from build123d import *

# Parameters (mm, degrees)
BOSS_EXTRUDE1_DEPTH = 3.175
SKETCH3_W           = 7.9375
SKETCH3_H           = 228.6
CUT_EXTRUDE1_DEPTH  = 184.546857096
SKETCH4_R           = 3.175
CUT_EXTRUDE2_DEPTH  = 184.546857096
SKETCH5_R           = 1.5
CUT_EXTRUDE3_DEPTH  = 3.175


with BuildPart() as part:
    # Sketch2 → Boss-Extrude1 (new body)
    with BuildSketch(Plane.XY):
        Polygon((-92.075, 152.4), (-92.075, 108.857142857), (-88.9, 108.857142857), (-88.9, 65.314285714), (-92.075, 65.314285714), (-92.075, 21.771428571), (-88.9, 21.771428571), (-88.9, -21.771428571), (-92.075, -21.771428571), (-92.075, -65.314285714), (-88.9, -65.314285714), (-88.9, -108.857142857), (-92.075, -108.857142857), (-92.075, -152.4), (-53.34, -152.4), (-53.34, -158.75), (-17.78, -158.75), (-17.78, -152.4), (17.78, -152.4), (17.78, -158.75), (53.34, -158.75), (53.34, -152.4), (92.075, -152.4), (92.075, -108.857142857), (88.9, -108.857142857), (88.9, -65.314285714), (92.075, -65.314285714), (92.075, -21.771428571), (88.9, -21.771428571), (88.9, 21.771428571), (92.075, 21.771428571), (92.075, 65.314285714), (88.9, 65.314285714), (88.9, 108.857142857), (92.075, 108.857142857), (92.075, 152.4), align=None)
    extrude(amount=BOSS_EXTRUDE1_DEPTH)

    # Sketch3 → Cut-Extrude1 (cut, through all)
    with BuildSketch(Plane.XY.offset(3.175)):
        with Locations((0, 38.1)):
            Rectangle(SKETCH3_W, SKETCH3_H)
    extrude(amount=-CUT_EXTRUDE1_DEPTH, mode=Mode.SUBTRACT)

    # Sketch4 → Cut-Extrude2 (cut, through all)
    with BuildSketch(Plane.XY.offset(3.175)):
        with Locations((-50.8, -139.7)):
            Circle(SKETCH4_R)
    extrude(amount=-CUT_EXTRUDE2_DEPTH, mode=Mode.SUBTRACT)

    # Sketch5 → Cut-Extrude3 (cut)
    with BuildSketch(Plane.XY.offset(3.175)):
        with Locations((-73.025, 122.4)):
            Circle(SKETCH5_R)
        with Locations((-73.025, 106.65)):
            Circle(SKETCH5_R)
        with Locations((73.025, 122.4)):
            Circle(SKETCH5_R)
        with Locations((73.025, 106.65)):
            Circle(SKETCH5_R)
    extrude(amount=-CUT_EXTRUDE3_DEPTH, mode=Mode.SUBTRACT)


solid = part.part
Build history of the part. All positions in model axes, mm. Coordinates: 2 decimals unless noted, no trailing zeros. Order: outer loops, then holes, each group sorted by start corner. A loop starts at its lowest first (then second) coordinate and runs counter-clockwise, first axis right, second up. Notation, with made-up numbers: M 36,-8 L 93,-8 A37 cw 93,28 Z; hole C 31.25,-14.75 d3. An arc over 180 degrees is marked long. One line per question, with ' | ' between items. Start each with the question number.
Q1. Saw through at B-B (y = 86). List the corners of the cut face in (x, z) (3 decimals).
Q2. Flat gauge pins, fed straight in: pin 1 Ø1 at (x, z) = (91, 1.5) entering from -Y; pin 2 Ø1.8 at (x, y) = (73.025, 106.65) entering from +Z; pin 3 Ø1 at (y, z) = (16, 1) entering from -X; pin 4 Ø1.5 at (y, z) = (73.5, 2) entering from +X. Where does each tip first touch, or does it go through?
Q3. Two-plate mould, pull along X, no slides. Class faces 1 (the face through (-22, -1, 3.175)), 2 (the face through (-51.21, -136.55, 1.61)): +X half, -X half, draft (parallel to the pull), parting line (faces both ways), or undercut.
Q4. Probe L1, parallel to X at y = 106.65, z = 1.65 (3 decimals); L2, parallel to X at y = 122.4, z = 2 (3 decimals); L3, parallel to X at y = -72.5, z = 0.55. List the from-to ranges inside material, lowest first. Write a range as from..to.
Q5. Saw through at C-C (z = 2.3). Count the separate pieces of the cut face and the enclosed holes in it, then the cut area to 3 significant figures.
Q6. Saw through at A-A (y = 42). List the corners of the cut face in (x, z) (3 decimals).
Q7. Saw through at D-D (x = 13.5). List the corners of the cut face in (y, z) (3 decimals), then the cut area to 3 significant figures.
Check values:
1) outline: M -88.9,0 L -3.969,0 L -3.969,3.175 L -88.9,3.175 Z; M 3.969,0 L 88.9,0 L 88.9,3.175 L 3.969,3.175 Z
2) pin 1: stops at y = -152.4 | pin 2: passes through | pin 3: stops at x = -88.9 | pin 4: stops at x = 88.9
3) face 1: draft | face 2: undercut
4) L1: x = -88.9..-74.525, -71.525..-3.969, 3.969..71.525, 74.525..88.9 | L2: x = -92.075..-74.525, -71.525..-3.969, 3.969..71.525, 74.525..92.075 | L3: x = -88.9..-3.97, 3.97..88.9
5) separate pieces: 1 | enclosed holes: 5 | area: 53,900 mm2
6) outline: M -92.075,0 L -3.969,0 L -3.969,3.175 L -92.075,3.175 Z; M 3.969,0 L 92.075,0 L 92.075,3.175 L 3.969,3.175 Z
7) outline: M -152.4,0 L 152.4,0 L 152.4,3.175 L -152.4,3.175 Z | area: 968 mm2
